Source: CAD feature listing. Evaluate the final solid. Frame: model axes, mm. A direction names the side the tool comes from. Give positions to 0.01 mm unless a question says otherwise; leave off trailing zeros. Write each loop counter-clockwise with the first axis right and the second up, starting at its lowest first coordinate (ties: lowest second). Pieces come first, ordered by that corner, then holes. Notation, with made-up numbers: M 33.25,80.5 L 79.25,80.5 A14 cw 79.25,84.5 Z; hole C 45,4.5 d7. An arc over 180 degrees is marked long. Use CSV: the item, a comma, the result in double quotes. Start each with the question number.
from build123d import *

# Parameters (mm, degrees)
F0_W     = 609.6
F0_H     = 457.2
F1_DEPTH = 304.8
F2_W     = 228.6
F2_H     = 355.6
F3_DEPTH = 6.35
F4_W     = 12.7
F4_H     = 127
F5_DEPTH = 12.7


with BuildPart() as f1:
    # F0 (on Front) → F1 (new body)
    with BuildSketch(Plane.XZ):
        with Locations((-27.527251, 34.139451)):
            Rectangle(F0_W, F0_H)
    extrude(amount=F1_DEPTH)

    # F2 (on face) → F3 (join)
    with BuildSketch(Plane.XZ.offset(304.8)):
        with Locations((-167.227251, 34.139451)):
            Rectangle(F2_W, F2_H)
        with Locations((112.172749, 34.139451)):
            Rectangle(F2_W, F2_H)
    extrude(amount=F3_DEPTH)

    # F4 (on face) → F5 (join)
    with BuildSketch(Plane.XZ.offset(311.15)):
        with Locations((-84.677251, -54.760549)):
            Rectangle(F4_W, F4_H)
        with Locations((29.622749, -54.760549)):
            Rectangle(F4_W, F4_H)
    extrude(amount=F5_DEPTH)


solid = f1.part
1. Pull-direction query (X, two-part tool) for faces 5 (the flat face through (-78.327, -317, -56)), 6 (the flat face through (-91.027, -317, -56)), 7 (the flat face through (-85, -317, 8.739)); classes: released by +X, released by -X, zero draft, split by the parting line, or undercut.
2. Section A-A on z = -46. Return loops of the section in (x, y).
3. Line query: probe 1 along X at (y, z) = (-305, 17.5); probe 2 along Y at (x, z) = (-144, 140); probe 3 along Y at (x, z) = (-28, 75.5). Output: solid intervals per line, ascending.
4. Section D-D on x = -43. Return loops of the section in (y, z), then the cut area to 3 significant figures.
5. First-contact query: pin 1 (5 mm diameter, centred on x = -145, y = -308, fed in from -Z); pin 2 (3 mm diameter, centred on x = -84, z = -146.5, fed in from +Y); pin 3 (14 mm diameter, centred on y = -319.5, z = -69, fed in from +X); pin 4 (3 mm diameter, centred on x = -118, y = -308.5, fed in from +Z). Flat tips, straight axial feed; report the tip coordinate or a pass-through.
6. Section C-C on z = 37. Return loops of the section in (x, y).
7. Section B-B on x = -236. Return loops of the section in (y, z).
8. Access query for faces 1 (the flat face through (30, -317, 8.739)), 2 (the flat face through (35.973, -317, -56)), 3 (the flat face through (-85, -317, -118.261)), 4 (the flat face through (23.273, -317, -56)). Directions: +Z, -Z, +X, -X, +Y, -Y. A direction counts if a zero-diameter tool reaches every point of the face in a straight line with its end or side. Return the directions, or none.
Resolved:
1,face 5,"undercut"
1,face 6,"released by -X"
1,face 7,"zero draft"
2,outline,"M -332.33,-304.8 L -281.53,-304.8 L -281.53,-311.15 L -91.03,-311.15 L -91.03,-323.85 L -78.33,-323.85 L -78.33,-311.15 L -52.93,-311.15 L -52.93,-304.8 L -2.13,-304.8 L -2.13,-311.15 L 23.27,-311.15 L 23.27,-323.85 L 35.97,-323.85 L 35.97,-311.15 L 226.47,-311.15 L 226.47,-304.8 L 277.27,-304.8 L 277.27,0 L -332.33,0 Z"
3,probe 1,"x = -281.53 to -52.93, -2.13 to 226.47"
3,probe 2,"y = -311.15 to 0"
3,probe 3,"y = -304.8 to 0"
4,outline,"M -304.8,-194.46 L 0,-194.46 L 0,262.74 L -304.8,262.74 Z"
4,area,"139,000 mm2"
5,pin 1,"stops at z = -143.66"
5,pin 2,"stops at y = 0"
5,pin 3,"stops at x = 35.97"
5,pin 4,"stops at z = 211.94"
6,outline,"M -332.33,-304.8 L -281.53,-304.8 L -281.53,-311.15 L -52.93,-311.15 L -52.93,-304.8 L -2.13,-304.8 L -2.13,-311.15 L 226.47,-311.15 L 226.47,-304.8 L 277.27,-304.8 L 277.27,0 L -332.33,0 Z"
7,outline,"M -311.15,-143.66 L -304.8,-143.66 L -304.8,-194.46 L 0,-194.46 L 0,262.74 L -304.8,262.74 L -304.8,211.94 L -311.15,211.94 Z"
8,face 1,"+Z, +X, -X, -Y"
8,face 2,"+Z, -Z, +X, -Y"
8,face 3,"-Z, +X, -X, -Y"
8,face 4,"+Z, -Z, -Y"
